from build123d import *

# Parameters (mm, degrees)
SKETCH1_W           = 700
SKETCH1_H           = 600
BOSS_EXTRUDE1_DEPTH = 30
SKETCH2_W           = 600
SKETCH2_H           = 700
BOSS_EXTRUDE2_DEPTH = 30
SKETCH3_W           = 600
SKETCH3_H           = 400
BOSS_EXTRUDE3_DEPTH = 700
SKETCH4_W           = 300
SKETCH4_H           = 20
BOSS_EXTRUDE4_DEPTH = 300


with BuildPart() as part:
    # Sketch1 → Boss-Extrude1 (new body)
    with BuildSketch(Plane(origin=(0, 0, 0), x_dir=(0, 1, 0), z_dir=(0, 0, 1))):
        Rectangle(SKETCH1_W, SKETCH1_H)
    extrude(amount=BOSS_EXTRUDE1_DEPTH)

    # Sketch2 → Boss-Extrude2 (add)
    with BuildSketch(Plane(origin=(0, 350, 0), x_dir=(-1, 0, 0), z_dir=(0, 1, 0))):
        with Locations((0, -320)):
            Rectangle(SKETCH2_W, SKETCH2_H)
    extrude(amount=BOSS_EXTRUDE2_DEPTH)

    # Sketch3 → Boss-Extrude3 (add)
    with BuildSketch(Plane.XY.offset(30)):
        with Locations((0, -550)):
            Rectangle(SKETCH3_W, SKETCH3_H)
    extrude(amount=-BOSS_EXTRUDE3_DEPTH)

    # Sketch4 → Boss-Extrude4 (add)
    with BuildSketch(Plane.XY.offset(30)):
        with Locations((-150, 370)):
            Rectangle(SKETCH4_W, SKETCH4_H)
    extrude(amount=BOSS_EXTRUDE4_DEPTH)


solid = part.part
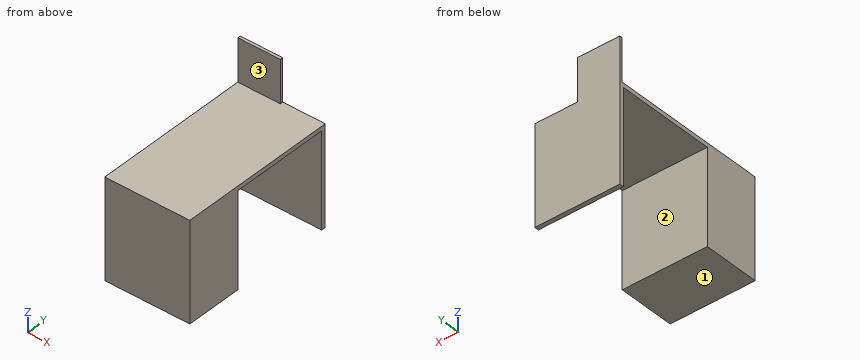
The model under review builds one solid part; all positions refer to its coordinate system, in mm. Face numbers are marked on the shaded views. A direction names the side the tool comes from. Round coordinates to 2 decimals unless told otherwise and drop trailing zeros. Write each loop counter-clockwise with the first axis right and the second up, starting at its lowest first coordinate (ties: lowest second). Pieces come first, ordered by that corner, then holes. Notation, with made-up numbers: M 29,56.5 L 86,56.5 A28 ccw 86,83.5 Z; hole C -39,75.25 d10. An arc over 180 degrees is marked long. Answer as CSV lines item,"result". Start each with the question number.
Q1. Consider section C-C, the plane y = 214. Give the boundary of the cut face in (x, z), then the cut area to 3 significant figures.
Q2. Consider section D-D, the plane z = 110.5. Give the boundary of the cut face in (x, y), then the cut area to 3 significant figures.
Q3. Consider section A-A, the plane z = -215. Give the boundary of the cut face in (x, y), then the cut area to 3 significant figures.
Q4. Consider section B-B, the plane x = -58.5. Give the boundary of the cut face in (y, z), then the cut area to 3 significant figures.
Q5. Clearance check with flat-ended pins moving along their axes: P1, Ø8, axis at x = 171.5, y = -333.5, coming from the -Z side; P2, Ø10, axis at y = 373.5, z = 249.5, coming from the +X side. State where each tip first meets the part, or that it passes through.
Q6. Wall thickness on line 1 along Y through (x, z) = (114, -409); line 2 along Z through (x, y) = (203, -280); line 3 along Y through (x, z) = (-89, 95.5): over which ranges is each line inside the solid? List them lowest first.
Q7. Tool access review of the marked faces 1, 2 and 3: name each direction out of +Z, -Z, +X, -X, +Y, -Y from which nothing blocks a thin tool from reaching the whole face with its end or side.
Result set:
1,outline,"M -300,0 L 300,0 L 300,30 L -300,30 Z"
1,area,"18,000 mm²"
2,outline,"M -300,360 L 0,360 L 0,380 L -300,380 Z"
2,area,"6,000 mm²"
3,outline,"M -300,-750 L 300,-750 L 300,-350 L -300,-350 Z; M -300,350 L 300,350 L 300,380 L -300,380 Z"
3,area,"258,000 mm²"
4,outline,"M -750,-670 L -350,-670 L -350,0 L 350,0 L 350,-670 L 380,-670 L 380,330 L 360,330 L 360,30 L -750,30 Z"
4,area,"328,000 mm²"
5,P1,"stops at z = 0"
5,P2,"stops at x = 0"
6,line 1,"y = -750 to -350, 350 to 380"
6,line 2,"z = 0 to 30"
6,line 3,"y = 360 to 380"
7,face 1,"-Z, +X, -X, +Y, -Y"
7,face 2,"-Z, +X, -X"
7,face 3,"+Z, +X, -X, -Y"
